Build history of the part. All positions in model axes, mm. Face numbers are marked on the shaded views. A direction names the side the tool comes from. Round coordinates to 2 decimals unless told otherwise and drop trailing zeros. Loops run counter-clockwise (first coordinate to the right, second up) from the corner with the lowest first, then second, coordinate; pieces in that order, holes last. Notation, with made-up numbers: (84.25, 28) -> (122.25, 28) arc R23 cw to (122.25, 67) -> close; hole circle Ø10 at (-10, 62). An arc over 180 degrees is marked (long way). Put each result on its own line as item: value. Start each with the question number.
Item 1: Cut at C-C, the plane y = -2.5. List the corners of the cut face in (x, z), plus the area to 3 significant figures.
Item 2: Cut at B-B, the plane z = 45.5. List the corners of the cut face in (x, y), plus the area to 3 significant figures.
Item 3: Drill centre lines: probe 1 along Y at (x, z) = (-446, 19.5); probe 2 along Z at (x, y) = (-452.5, -6); probe 3 along Y at (x, z) = (-461.5, 6.5). Where is each one in solid material? Low to high. Write a range as [from, to].
Item 4: Tool access for the marked faces 5 and 6: list every direction of +Z, -Z, +X, -X, +Y, -Y with a clear straight run to the whole face (end or side of a thin tool).
Item 5: Pull direction Y, two halves, no side cores. Call the marked faces 1, 2, 3 and 4: +Y half, -Y half, draft (parallel to the pull), parting line (faces both ways), or undercut.
Item 6: Cut at A-A, the plane x = -446.5. List the corners of the cut face in (y, z), plus the area to 3 significant figures.
Item 7: Cut at D-D, the plane x = -426.5. Count the separate pieces of the cut face and the enclosed holes in it, plus the area to 3 significant figures.
Item 8: Flat gauge pin, fed straight in: pin 1 Ø3 at (x, y) = (-460.88, 5.63) entering from +Z. Where does the tip first touch, or does it go through?
```python
from build123d import *

# Parameters (mm, degrees)
SKETCH1_W               = 50
SKETCH1_H               = 40
BOSS_EXTRUDE1_DEPTH     = 4
SKETCH2_W               = 50
SKETCH2_H               = 4
BOSS_EXTRUDE2_DEPTH     = 55.38
SKETCH4_W               = 50
SKETCH4_H               = 4
BOSS_EXTRUDE3_DEPTH     = 32
SKETCH5_R               = 1.6
CUT_EXTRUDE1_DEPTH      = 1
CUT_EXTRUDE1_DEPTH_BACK = 60.38
CUT_EXTRUDE2_START      = -2
CUT_EXTRUDE2_DEPTH      = 55.38
FILLET1_R               = 6


with BuildPart() as part:
    # Sketch1 → Boss-Extrude1 (new body)
    with BuildSketch(Plane.XY):
        with Locations((-443.882332823, -0.367507575)):
            Rectangle(SKETCH1_W, SKETCH1_H)
    extrude(amount=BOSS_EXTRUDE1_DEPTH)

    # Sketch2 → Boss-Extrude2 (add)
    with BuildSketch(Plane.XY.offset(4)):
        with Locations((-443.882332823, -18.367507575)):
            Rectangle(SKETCH2_W, SKETCH2_H)
        with Locations((-443.882332823, 17.632492425)):
            Rectangle(SKETCH2_W, SKETCH2_H)
    extrude(amount=BOSS_EXTRUDE2_DEPTH)

    # Sketch4 → Boss-Extrude3 (add)
    with BuildSketch(Plane.XZ.offset(-15.632492425)):
        with Locations((-443.882332823, 57.38)):
            Rectangle(SKETCH4_W, SKETCH4_H)
    extrude(amount=BOSS_EXTRUDE3_DEPTH)

    # Sketch5 → Cut-Extrude1 (cut, two sides)
    with BuildSketch(Plane.XY.offset(59.38)) as cut_extrude1_sk:
        with Locations((-460.882332823, -6.367507575)):
            Circle(SKETCH5_R)
        with Locations((-460.882332823, 5.632492425)):
            Circle(SKETCH5_R)
        with Locations((-426.882332823, -6.367507575)):
            Circle(SKETCH5_R)
        with Locations((-426.882332823, 5.632492425)):
            Circle(SKETCH5_R)
    extrude(amount=CUT_EXTRUDE1_DEPTH, mode=Mode.SUBTRACT)
    extrude(cut_extrude1_sk.sketch, amount=-CUT_EXTRUDE1_DEPTH_BACK, mode=Mode.SUBTRACT)

    # Sketch6 → Cut-Extrude2 (cut)
    with BuildSketch(Plane(origin=(0, 0, 55.38), x_dir=(-1, 0, 0), z_dir=(0, 0, -1)).offset(CUT_EXTRUDE2_START)):
        Polygon((457.620303802, 5.632492425), (459.251318313, 2.807492425), (462.513347334, 2.807492425), (464.144361844, 5.632492425), (462.513347334, 8.457492425), (459.251318313, 8.457492425), align=None)
        Polygon((457.620303802, -6.367507575), (459.251318313, -9.192507575), (462.513347334, -9.192507575), (464.144361844, -6.367507575), (462.513347334, -3.542507575), (459.251318313, -3.542507575), align=None)
        Polygon((425.251318313, 2.807492425), (428.513347334, 2.807492425), (430.144361844, 5.632492425), (428.513347334, 8.457492425), (425.251318313, 8.457492425), (423.620303802, 5.632492425), align=None)
        Polygon((423.620303802, -6.367507575), (425.251318313, -9.192507575), (428.513347334, -9.192507575), (430.144361844, -6.367507575), (428.513347334, -3.542507575), (425.251318313, -3.542507575), align=None)
    extrude(amount=CUT_EXTRUDE2_DEPTH, mode=Mode.SUBTRACT)

    # Fillet1
    fillet1_edges = [part.edges().sort_by_distance(p)[0] for p in [
        (-443.882332823, -16.367507575, 4),
        (-443.882332823, 15.632492425, 4),
        (-443.882332823, 15.632492425, 55.38),
        (-443.882332823, -16.367507575, 55.38),
    ]]
    fillet(fillet1_edges, radius=FILLET1_R)


solid = part.part
```
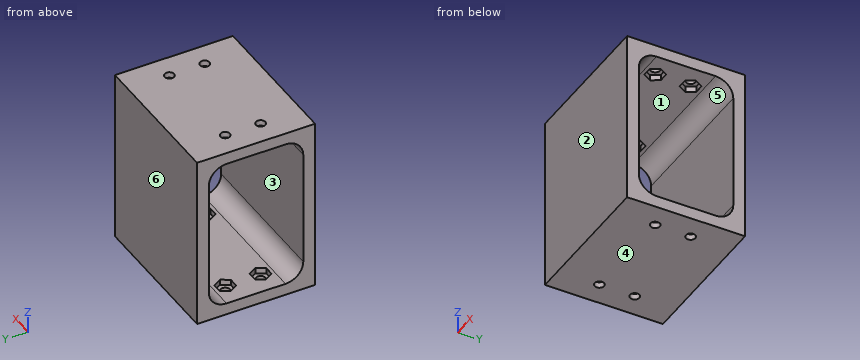
Reply:
1. outline: (-468.88, 0) -> (-418.88, 0) -> (-418.88, 4) -> (-468.88, 4) -> close; (-468.88, 55.38) -> (-418.88, 55.38) -> (-418.88, 59.38) -> (-468.88, 59.38) -> close
1. area: 400 mm^2
2. outline: (-468.88, -20.37) -> (-418.88, -20.37) -> (-418.88, -16.37) -> (-468.88, -16.37) -> close; (-468.88, 15.63) -> (-418.88, 15.63) -> (-418.88, 19.63) -> (-468.88, 19.63) -> close
2. area: 400 mm^2
3. probe 1: y = [-20.37, -16.37], [15.63, 19.63]
3. probe 2: z = [0, 4], [55.38, 59.38]
3. probe 3: y = [-20.37, -15.24], [14.51, 19.63]
4. face 5: +X, -X
4. face 6: +Z, -Z, +X, -X, +Y
5. face 1: undercut
5. face 2: -Y half
5. face 3: undercut
5. face 4: draft
6. outline: (-20.37, 0) -> (19.63, 0) -> (19.63, 59.38) -> (-20.37, 59.38) -> close; hole (-16.37, 10) arc R6 ccw to (-10.37, 4) -> (9.63, 4) arc R6 ccw to (15.63, 10) -> (15.63, 49.38) arc R6 ccw to (9.63, 55.38) -> (-10.37, 55.38) arc R6 ccw to (-16.37, 49.38) -> close
6. area: 762 mm^2
7. separate pieces: 4
7. enclosed holes: 0
7. area: 692 mm^2
8. pin 1: passes through
